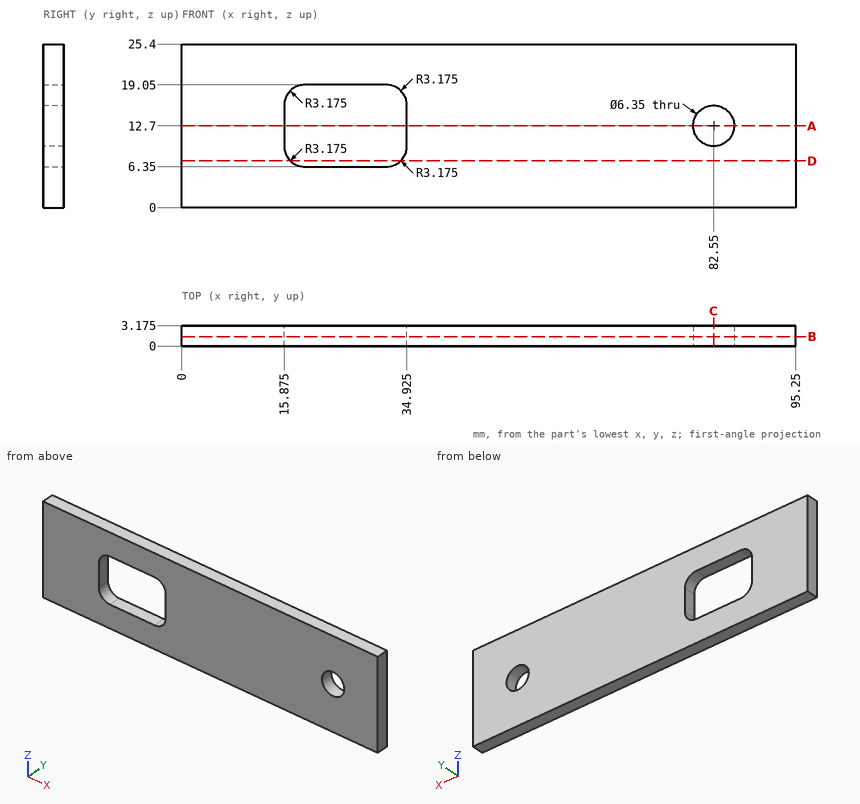
Input: dimensioned drawing with shaded views. Units: mm. Origin: part minimum x, y, z. Round coordinates to 2 decimals unless told otherwise and drop trailing zeros. Loops run counter-clockwise (first coordinate to the right, second up) from the corner with the lowest first, then second, coordinate; pieces in that order, holes last. Notation, with made-up numbers: M 26,4.5 L 79,4.5 A10 cw 79,12.5 Z; hole C 45.5,-4 d11. An arc over 180 degrees is marked long. One line per question, with ' | ' between items.
(1) Cut plane A-A on z = 12.7. Return the cut outline in (x, y) (3 decimals), plus the area to 3 significant figures.
Check result:
outline: M 0,0 L 15.875,0 L 15.875,3.175 L 0,3.175 Z; M 34.925,0 L 79.375,0 L 79.375,3.175 L 34.925,3.175 Z; M 85.725,0 L 95.25,0 L 95.25,3.175 L 85.725,3.175 Z | area: 222 mm2
(2) Contact query for a flat-ended pin moving along its axis: P1, Ø4, axis at x = 23.5, z = 10, coming from the +Y side. Output: stop coordinate, or through.
Check result:
P1: passes through
(3) Cut plane D-D on z = 7.25. Return the cut outline in (x, y) (3 decimals).
Check result:
outline: M 0,0 L 16.835,0 L 16.835,3.175 L 0,3.175 Z; M 33.965,0 L 95.25,0 L 95.25,3.175 L 33.965,3.175 Z
(4) Cut plane B-B on y = 1.45. Return the cut outline in (x, z) (3 decimals).
Check result:
outline: M 0,0 L 95.25,0 L 95.25,25.4 L 0,25.4 Z; hole M 15.875,9.525 A3.175 ccw 19.05,6.35 L 31.75,6.35 A3.175 ccw 34.925,9.525 L 34.925,15.875 A3.175 ccw 31.75,19.05 L 19.05,19.05 A3.175 ccw 15.875,15.875 Z; hole C 82.55,12.7 d6.35
(5) Material intervals for line 1 along X through (y, z) = (1.15, 12.7) (3 decimals); line 2 along Z through (x, y) = (31, 2.1); line 3 along X through (y, z) = (1.8, 13.75) (3 decimals), sorted ascending. Write a range as from..to.
Check result:
line 1: x = 0..15.875, 34.925..79.375, 85.725..95.25 | line 2: z = 0..6.35, 19.05..25.4 | line 3: x = 0..15.875, 34.925..79.554, 85.546..95.25
(6) Cut plane C-C on x = 82.55. Return the cut outline in (y, z) (3 decimals).
Check result:
outline: M 0,0 L 3.175,0 L 3.175,9.525 L 0,9.525 Z; M 0,15.875 L 3.175,15.875 L 3.175,25.4 L 0,25.4 Z
